from build123d import *

# Parameters (mm, degrees)
SKETCH1_W               = 38.1
SKETCH1_H               = 38.1
BOSS_EXTRUDE1_DEPTH     = 50.8
SKETCH2_W               = 17.78
SKETCH2_H               = 18.288
BOSS_EXTRUDE2_DEPTH     = 50.8
SKETCH3_R               = 19.05
BOSS_EXTRUDE3_DEPTH     = 12.7
SKETCH4_W               = 17.78
SKETCH4_H               = 18.288
BOSS_EXTRUDE4_DEPTH     = 137.16
SKETCH6_R               = 12.7
BOSS_EXTRUDE5_DEPTH     = 31.75
SKETCH7_R               = 5.08
CUT_EXTRUDE1_DEPTH      = 63.5
SKETCH8_R               = 1.27
CUT_EXTRUDE2_DEPTH      = 10.16
SKETCH8_3_R             = 1.27
CUT_EXTRUDE3_DEPTH      = 10.16
SKETCH8_4_R             = 1.27
CUT_EXTRUDE4_DEPTH      = 10.16
SKETCH8_5_R             = 1.27
CUT_EXTRUDE5_DEPTH      = 10.16
FILLET1_R               = 6.35
SKETCH10_R              = 1.905
CUT_EXTRUDE6_DEPTH      = 2.54
MIRROR2_COPY_1_SKETCH_R = 1.905
MIRROR2_COPY_1_DEPTH    = 2.54
FILLET2_R               = 2.54


with BuildPart() as part:
    # Sketch1 → Boss-Extrude1 (new body)
    with BuildSketch(Plane.XY):
        Rectangle(SKETCH1_W, SKETCH1_H)
    extrude(amount=BOSS_EXTRUDE1_DEPTH)

    # Sketch2 → Boss-Extrude2 (add)
    with BuildSketch(Plane.XY.offset(50.8)):
        Rectangle(SKETCH2_W, SKETCH2_H)
    extrude(amount=BOSS_EXTRUDE2_DEPTH)

    # Sketch3 → Boss-Extrude3 (add)
    with BuildSketch(Plane.XY.offset(101.6)):
        Circle(SKETCH3_R)
    extrude(amount=BOSS_EXTRUDE3_DEPTH)

    # Sketch4 → Boss-Extrude4 (add)
    with BuildSketch(Plane(origin=(0, 19.05, 0), x_dir=(1, 0, 0), z_dir=(0, 1, 0))):
        with Locations((0, -25.4)):
            Rectangle(SKETCH4_W, SKETCH4_H)
    extrude(amount=BOSS_EXTRUDE4_DEPTH)

    # Sketch6 → Boss-Extrude5 (add, symmetric)
    with BuildSketch(Plane(origin=(0, 0, 0), x_dir=(0, 0, -1), z_dir=(1, 0, 0))):
        with Locations((-25.4, 163.83)):
            Circle(SKETCH6_R)
    extrude(amount=BOSS_EXTRUDE5_DEPTH, both=True)

    # Sketch7 → Cut-Extrude1 (cut)
    with BuildSketch(Plane(origin=(31.75, 0, 0), x_dir=(0, 0, -1), z_dir=(1, 0, 0))):
        with Locations((-25.4, 163.83)):
            Circle(SKETCH7_R)
    extrude(amount=-CUT_EXTRUDE1_DEPTH, mode=Mode.SUBTRACT)

    # Sketch8 → Cut-Extrude2 (cut)
    with BuildSketch(Plane.XY.offset(114.3)):
        with Locations((8.89, 9.144)):
            Circle(SKETCH8_R)
    extrude(amount=-CUT_EXTRUDE2_DEPTH, mode=Mode.SUBTRACT)

    # Sketch8_3 → Cut-Extrude3 (cut)
    with BuildSketch(Plane.XY.offset(114.3)):
        with Locations((8.89, -9.144)):
            Circle(SKETCH8_3_R)
    extrude(amount=-CUT_EXTRUDE3_DEPTH, mode=Mode.SUBTRACT)

    # Sketch8_4 → Cut-Extrude4 (cut)
    with BuildSketch(Plane.XY.offset(114.3)):
        with Locations((-8.89, -9.144)):
            Circle(SKETCH8_4_R)
    extrude(amount=-CUT_EXTRUDE4_DEPTH, mode=Mode.SUBTRACT)

    # Sketch8_5 → Cut-Extrude5 (cut)
    with BuildSketch(Plane.XY.offset(114.3)):
        with Locations((-8.89, 9.144)):
            Circle(SKETCH8_5_R)
    extrude(amount=-CUT_EXTRUDE5_DEPTH, mode=Mode.SUBTRACT)

    # Fillet1
    fillet1_edges = [part.edges().sort_by_distance(p)[0] for p in [
        (0, 19.05, 50.8),
        (-8.89, -9.144, 76.2),
        (8.89, -9.144, 76.2),
        (-19.05, 0, 50.8),
        (8.89, 9.144, 76.2),
        (-8.89, 9.144, 76.2),
        (-8.89, 87.0332647, 34.544),
        (-8.89, 87.0332647, 16.256),
        (8.89, 87.0332647, 16.256),
        (8.89, 87.0332647, 34.544),
        (0, -19.05, 50.8),
        (-19.05, 0, 0),
        (0, 19.05, 0),
        (19.05, 0, 0),
        (0, -19.05, 0),
        (-19.05, -19.05, 25.4),
        (-19.05, 19.05, 25.4),
        (19.05, 19.05, 25.4),
        (19.05, -19.05, 25.4),
        (19.05, 0, 50.8),
    ]]
    fillet(fillet1_edges, radius=FILLET1_R)

    # Sketch10 → Cut-Extrude6 (cut)
    with BuildSketch(Plane.XY.offset(104.14)):
        with Locations((-8.89, -9.144)):
            Circle(SKETCH10_R)
    cut_extrude6 = extrude(amount=-CUT_EXTRUDE6_DEPTH, mode=Mode.SUBTRACT)

    # Mirror1: Cut-Extrude6 across plane
    add(cut_extrude6.mirror(Plane.ZX), mode=Mode.SUBTRACT)

    # Mirror2: Cut-Extrude6 across plane
    add(cut_extrude6.mirror(Plane(origin=(0, 0, 0), x_dir=(0, 0, 1), z_dir=(1, 0, 0))), mode=Mode.SUBTRACT)

    # Mirror2 copy 1 sketch → Mirror2 copy 1 (cut)
    with BuildSketch(Plane(origin=(0, 0, 104.14), x_dir=(-1, 0, 0), z_dir=(0, 0, 1))):
        with Locations((-8.89, -9.144)):
            Circle(MIRROR2_COPY_1_SKETCH_R)
    extrude(amount=-MIRROR2_COPY_1_DEPTH, mode=Mode.SUBTRACT)

    # Fillet2
    fillet2_edges = [part.edges().sort_by_distance(p)[0] for p in [
        (-19.05, 0, 101.6),
    ]]
    fillet(fillet2_edges, radius=FILLET2_R)


solid = part.part
Geometry: final body of the model. Coordinates: model frame, mm. A direction names the side the tool comes from. Give positions to 0.01 mm unless a question says otherwise; leave off trailing zeros. Write each loop counter-clockwise with the first axis right and the second up, starting at its lowest first coordinate (ties: lowest second). Pieces come first, ordered by that corner, then holes. Notation, with made-up numbers: M 50.25,61 L 59.25,61 A22 ccw 59.25,82 Z; hole C 35,0.25 d5. An arc over 180 degrees is marked long. Answer in a Markdown table with one row per item. Add a question column.
(1) First-contact query: pin 1 (3 mm diameter, centred on y = 67, z = 26.5, fed in from +X); pin 2 (1.5 mm diameter, centred on x = -8.89, y = -9.144, fed in from +Z); pin 3 (7.5 mm diameter, centred on y = -4, z = 33, fed in from +X). Flat tips, straight axial feed; report the tip coordinate or a pass-through.
(2) Mould query, pull axis Z, two halves, no side actions, for faces 1 (the flat face through (8.89, 0, 76)), 2 (the cylindrical face through (17.14, 0.18, 1.81)), 3 (the cylindrical face through (17.24, -17.14, 25.67)), 4 (the cylindrical face through (0.444, 176.422, 27.053)). Classes: +Z half, -Z half, draft (parallel to the pull), parting line (faces both ways), or undercut.
(3) Reachability of faces 5 (the flat face through (0, 86, 34.544)), 6 (the flat face through (-8.89, 0, 76)), 7 (the cylindrical face through (6.98, -7.333, 76.556)), 8 (the cylindrical face through (-17.14, 17.24, 25.67)), 9 (the cylindrical face through (7.079, 7.234, 76.556)) from +Z, -Z, +X, -X, +Y, -Y: full face, straight path, thin tool, end or side. Return the list, or none.
(4) Section A-A on x = 0. Return loops of the section in (y, z).
(5) Section D-D on z = 94.5. Return loops of the section in (x, y), and give its area (3 significant figures).
(6) Section C-C on y = 77. Return loops of the section in (x, z), and give its area (3 significant figures).
(7) Section B-B on y = 163.83. Return loops of the section in (x, z).
(8) Ray query, line 1 (Y direction, x = 4, z = 25); line 2 (Y direction, x = 8.89, z = 103.5); line 3 (Y direction, x = -8.89, z = 107.5). Return the intervals inside material, ascending.
Result set:
| question | item | result |
|---|---|---|
| 1 | pin 1 | stops at x = 8.89 |
| 1 | pin 2 | stops at z = 50.8 |
| 1 | pin 3 | stops at x = 19.05 |
| 2 | face 1 | undercut |
| 2 | face 2 | -Z half |
| 2 | face 3 | draft |
| 2 | face 4 | parting line |
| 3 | face 5 | +Z, +X, -X |
| 3 | face 6 | -X, +Y, -Y |
| 3 | face 7 | +X, -Y |
| 3 | face 8 | +Z, -Z, -X |
| 3 | face 9 | +X, +Y |
| 4 | outline | M -19.05,6.35 A6.35 ccw -12.7,0 L 12.7,0 A6.35 ccw 19.05,6.35 L 19.05,16.26 L 155.02,16.26 A12.7 ccw long 155.02,34.54 L 19.05,34.54 L 19.05,44.45 A6.35 ccw 12.7,50.8 L 9.14,50.8 L 9.14,101.6 L 16.51,101.6 A2.54 ccw 19.05,104.14 L 19.05,114.3 L -19.05,114.3 L -19.05,104.14 A2.54 ccw -16.51,101.6 L -9.14,101.6 L -9.14,50.8 L -12.7,50.8 A6.35 ccw -19.05,44.45 Z; hole C 163.83,25.4 d10.16 |
| 5 | outline | M -8.89,-2.79 A6.35 ccw -2.54,-9.14 L 2.54,-9.14 A6.35 ccw 8.89,-2.79 L 8.89,2.79 A6.35 ccw 2.54,9.14 L -2.54,9.14 A6.35 ccw -8.89,2.79 Z |
| 5 | area | 291 mm^2 |
| 6 | outline | M -8.89,22.61 A6.35 ccw -2.54,16.26 L 2.54,16.26 A6.35 ccw 8.89,22.61 L 8.89,28.19 A6.35 ccw 2.54,34.54 L -2.54,34.54 A6.35 ccw -8.89,28.19 Z |
| 6 | area | 291 mm^2 |
| 7 | outline | M -31.75,12.7 L 31.75,12.7 L 31.75,20.32 L -31.75,20.32 Z; M -31.75,30.48 L 31.75,30.48 L 31.75,38.1 L -31.75,38.1 Z |
| 8 | line 1 | y = -19.05 to 158.77, 168.89 to 176.52 |
| 8 | line 2 | y = -16.76 to -11.05, -7.24 to 7.24, 11.05 to 16.76 |
| 8 | line 3 | y = -16.85 to -10.41, -7.87 to 7.87, 10.41 to 16.85 |
